Source: CAD feature listing. Evaluate the final solid. Frame: model axes, mm. Face numbers are marked on the shaded views. A direction names the side the tool comes from. Give positions to 0.01 mm unless a question says otherwise; leave off trailing zeros. Write each loop counter-clockwise with the first axis right and the second up, starting at its lowest first coordinate (ties: lowest second). Pieces come first, ordered by that corner, then holes. Notation, with made-up numbers: M 42.5,5 L 71.5,5 A15 ccw 71.5,32 Z; hole C -11.75,-28 d5. An arc over 180 degrees is marked long. Return JSON: item names as keys, results as strings.
```python
from build123d import *

# Parameters (mm, degrees)
BOSS_EXTRUDE1_DEPTH = 9
SKETCH3_OUTSIDE_W   = 13.486
SKETCH3_OUTSIDE_H   = 12.496
SKETCH3_OUTSIDE_R   = 3.2
CUT_EXTRUDE1_DEPTH  = 1


with BuildPart() as part:
    # Sketch1 → Boss-Extrude1 (new, symmetric)
    with BuildSketch(Plane(origin=(0, 0, 0), x_dir=(1, 0, 0), z_dir=(0, 1, 0))):
        Polygon((3.695041723, 0), (1.847520861, 3.2), (-1.847520861, 3.2), (-3.695041723, 0), (-1.847520861, -3.2), (1.847520861, -3.2), align=None)
    extrude(amount=BOSS_EXTRUDE1_DEPTH, both=True)

    # Sketch3 outside → Cut-Extrude1 (cut)
    with BuildSketch(Plane(origin=(0, 9, 0), x_dir=(1, 0, 0), z_dir=(0, 1, 0))):
        Rectangle(SKETCH3_OUTSIDE_W, SKETCH3_OUTSIDE_H)
        with Locations(Location((0, 0, 0), (0, 0, 270))):
            Circle(SKETCH3_OUTSIDE_R, mode=Mode.SUBTRACT)
    cut_extrude1 = extrude(amount=-CUT_EXTRUDE1_DEPTH, mode=Mode.SUBTRACT)

    # Mirror2: Cut-Extrude1 across plane
    add(cut_extrude1.mirror(Plane.ZX), mode=Mode.SUBTRACT)

    # Sketch2 → M2.5 Tapped Hole1 (revolve, cut)
    with BuildSketch(Plane(origin=(0, 9, 0), x_dir=(0, 0, 1), z_dir=(1, 0, 0))):
        Polygon((0, 0), (0, 6.965882135), (1.025, 6.35), (1.025, 0), align=None)
    m2_5_tapped_hole1 = revolve(axis=Axis((0, 15.35, 0), (0, -1, 0)), mode=Mode.SUBTRACT)

    # Mirror1: M2.5 Tapped Hole1 across plane
    add(m2_5_tapped_hole1.mirror(Plane.ZX), mode=Mode.SUBTRACT)


solid = part.part
```
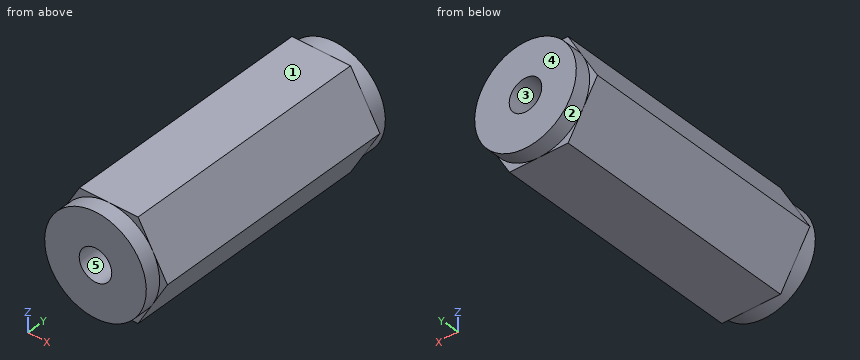
1) Set-up query: the marked faces 4 and 5. Return all of +Z, -Z, +X, -X, +Y, -Y with unobstructed straight access to the full face (end or side cutting, diameter ignored); none if empty.
Numbers:
{"face 4": "+Z, -Z, +X, -X, +Y", "face 5": "-Y"}
2) Cut plane A-A, the plane y = -7.5. Return the cut outline in (x, z) (3 decimals).
Numbers:
{"outline": "M -3.695,0 L -1.848,-3.2 L 1.848,-3.2 L 3.695,0 L 1.848,3.2 L -1.848,3.2 Z; hole C 0,0 d2.05"}
3) Line query: line 1 (Z direction, x = -0.5, y = -5); line 2 (X direction, y = 0.25, z = 2.5); line 3 (X direction, y = 0.25, z = 1). Output: solid intervals per line, ascending. Write a range as [from, to].
Numbers:
{"line 1": "z = [-3.2, -0.89], [0.89, 3.2]", "line 2": "x = [-2.25, 2.25]", "line 3": "x = [-3.12, 3.12]"}
4) Cut plane B-B, the plane x = 3. Return the cut outline in (y, z).
Numbers:
{"outline": "M -9,-1.11 L -8,-1.11 L -8,-1.2 L 8,-1.2 L 8,-1.11 L 9,-1.11 L 9,1.11 L 8,1.11 L 8,1.2 L -8,1.2 L -8,1.11 L -9,1.11 Z"}
5) Draft query along Z for the marked faces 1, 2 and 3. Return one class per face: released by +Z, released by -Z, zero draft, split by the parting line, or undercut.
Numbers:
{"face 1": "released by +Z", "face 2": "split by the parting line", "face 3": "undercut"}
6) Cut plane C-C, the plane z = 2.5. Return the cut outline in (x, y), then the cut area to 3 significant figures.
Numbers:
{"outline": "M -2.25,-8 L -2,-8 L -2,-9 L 2,-9 L 2,-8 L 2.25,-8 L 2.25,8 L 2,8 L 2,9 L -2,9 L -2,8 L -2.25,8 Z", "area": "80.0 mm²"}
7) Cut plane D-D, the plane y = 1. Return the cut outline in (x, z), then the cut area to 3 significant figures.
Numbers:
{"outline": "M -3.7,0 L -1.85,-3.2 L 1.85,-3.2 L 3.7,0 L 1.85,3.2 L -1.85,3.2 Z", "area": "35.5 mm²"}
8) Contact query for flat-ended pins moving along their axis: pin 1 Ø3 at (y, z) = (0, -2.5) entering from -X; pin 2 Ø1.2 at (x, z) = (0, 0) entering from +Y; pin 3 Ø1.2 at (x, z) = (0, 0) entering from -Y; pin 4 Ø0.7 at (x, z) = (-3.5, 0) entering from -Y. Output: stop coordinate, or through.
Numbers:
{"pin 1": "stops at x = -3.12", "pin 2": "stops at y = 2.39", "pin 3": "stops at y = -2.39", "pin 4": "stops at y = -9"}
